from build123d import *

# Parameters (mm, degrees)
F0_R     = 25.4
F0_R_2   = 6.35
F1_DEPTH = 25.4
F2_R     = 5.08
F3_DEPTH = 25.4


with BuildPart() as f1:
    # F0 (on Front) → F1 (new body)
    with BuildSketch(Plane.XZ):
        Circle(F0_R)
        Circle(F0_R_2, mode=Mode.SUBTRACT)
        Circle(F0_R_2)
    extrude(amount=F1_DEPTH)

    # F2
    f2_edges = [f1.edges().sort_by_distance(p)[0] for p in [
        (-25.4, -25.4, 0),
        (-25.4, 0, 0),
    ]]
    fillet(f2_edges, radius=F2_R)

    # F0 (on Front) → F3 (join)
    with BuildSketch(Plane.XZ):
        Circle(F0_R_2)
    extrude(amount=-F3_DEPTH)


solid = f1.part
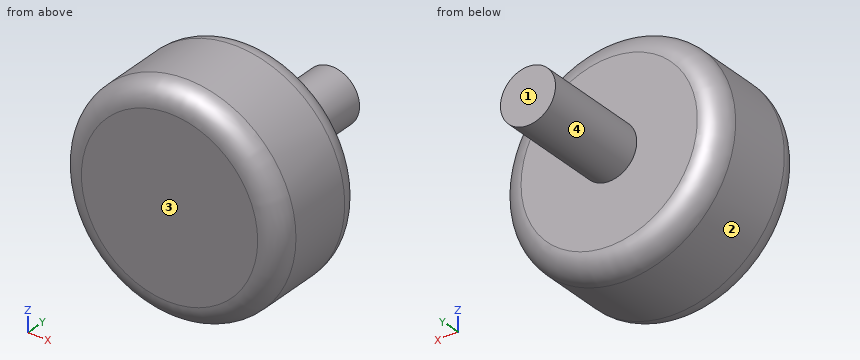
Verification items for the finished model (mm, model axes). Face numbers are marked on the shaded views. A direction names the side the tool comes from. Coordinates: 2 decimals unless noted, no trailing zeros. Order: outer loops, then holes, each group sorted by start corner. A loop starts at its lowest first (then second) coordinate and runs counter-clockwise, first axis right, second up. Notation, with made-up numbers: M 6.5,-1 L 52.5,-1 A23 cw 52.5,37 Z; hole C -35.5,69 d2. An arc over 180 degrees is marked long. One line per item, written item: value. Start each with the question number.
Item 1: Thickness scan on probe 1 along Y at (x, z) = (-19, 3); probe 2 along Z at (x, y) = (1.5, 6.5); probe 3 along X at (y, z) = (-2, 22.5). Record the ranges inside material, lowest first.
Item 2: Sectioned sample at D-D on y = -3. Record the cut outline in (x, z), then the cut area to 3 significant figures.
Item 3: Depth check by flat-ended pin: P1, Ø10, axis at x = -18, y = 3.5, coming from the -Z side; P2, Ø3, axis at x = 17.5, z = 10, coming from the +Y side; P3, Ø10, axis at y = 18, z = -1.5, coming from the -X side. Enter the tip coordinate at first touch or a pass-through.
Item 4: Mould release check, pull along Z, two halves, no side actions. Record for the marked faces 1 and 2: pulls with the +Z half, pulls with the -Z half, needs draft (parallel to the pull), parting line crosses it, or undercut.
Item 5: Sectioned sample at C-C on y = 3. Record the cut outline in (x, z), then the cut area to 3 significant figures.
Item 6: Sectioned sample at A-A on x = 0. Record the cut outline in (y, z).
Item 7: Access from +Z, -Z, +X, -X, +Y, -Y to the whole of each face (thin tool, end or side, straight path). Record for the marked faces 3 and 4.
Item 8: Sectioned sample at B-B on z = 0. Record the cut outline in (x, y), then the cut area to 3 significant figures.
Calculated:
1. probe 1: -25.4 to 0
1. probe 2: -6.17 to 6.17
1. probe 3: -9.34 to 9.34
2. outline: C 0,0 d49.91
2. area: 1,960 mm^2
3. P1: z = -17.17
3. P2: y = 0
3. P3: x = -6.35
4. face 1: needs draft
4. face 2: parting line crosses it
5. outline: C 0,0 d12.7
5. area: 127 mm^2
6. outline: M -25.4,-20.32 A5.08 ccw -20.32,-25.4 L -5.08,-25.4 A5.08 ccw 0,-20.32 L 0,-6.35 L 25.4,-6.35 L 25.4,6.35 L 0,6.35 L 0,20.32 A5.08 ccw -5.08,25.4 L -20.32,25.4 A5.08 ccw -25.4,20.32 Z
7. face 3: +Z, -Z, +X, -X, -Y
7. face 4: +Y
8. outline: M -25.4,-20.32 A5.08 ccw -20.32,-25.4 L 20.32,-25.4 A5.08 ccw 25.4,-20.32 L 25.4,-5.08 A5.08 ccw 20.32,0 L 6.35,0 L 6.35,25.4 L -6.35,25.4 L -6.35,0 L -20.32,0 A5.08 ccw -25.4,-5.08 Z
8. area: 1,590 mm^2
